Work out the finished part from the listing and answer in its coordinate system (mm). Face numbers are marked on the shaded views. A direction names the side the tool comes from. Coordinates: 2 decimals unless noted, no trailing zeros. Order: outer loops, then holes, each group sorted by start corner. A loop starts at its lowest first (then second) coordinate and runs counter-clockwise, first axis right, second up. Notation, with made-up numbers: M 78.25,-18.5 L 131.25,-18.5 A17 ccw 131.25,-3.5 Z; hole C -27,-6.75 d4. An arc over 180 degrees is marked long. Use a Markdown table: item, result.
from build123d import *

# Parameters (mm, degrees)
F0_W     = 430
F0_H     = 80
F1_DEPTH = 40
F2_W     = 7
F2_H     = 17.641502
F3_DEPTH = 30


with BuildPart() as f1:
    # F0 (on Right) → F1 (new body, symmetric)
    with BuildSketch(Plane.YZ):
        Rectangle(F0_W, F0_H)
    extrude(amount=F1_DEPTH, both=True)

    # F2 (on Right) → F3 (cut, symmetric)
    with BuildSketch(Plane.YZ):
        with Locations((-88.5, -48.820751)):
            Rectangle(F2_W, F2_H)
        Polygon((-92, -40), (-85, -40), (-17.87203, 40), (-17.87203, 50), (-106.093367, 50), (-106.093367, 40), (-87.336923, -30), align=None)
    extrude(amount=F3_DEPTH, both=True, mode=Mode.SUBTRACT)


solid = f1.part
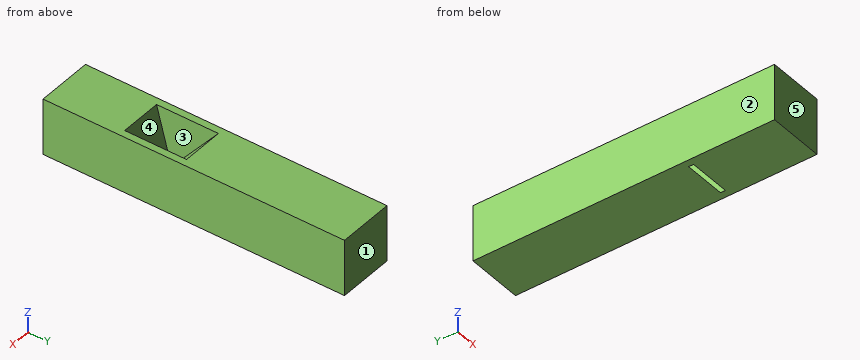
1. Section A-A on x = 12 is taken. Determine the outline of the cut face in (y, z), then the cut area to 3 significant figures.
Answers below:
| item | result |
|---|---|
| outline | M -215,-40 L -92,-40 L -87.34,-30 L -106.09,40 L -215,40 Z; M -85,-40 L 215,-40 L 215,40 L -17.87,40 Z |
| area | 30,800 mm² |
2. Find the intervals of material crossed by probe 1 along X at (y, z) = (-50.5, 8.5); probe 2 along Y at (x, z) = (-13, -10); probe 3 along Y at (x, z) = (16, 25.5), in increasing order.
Answers below:
| item | result |
|---|---|
| probe 1 | -40 to -30, 30 to 40 |
| probe 2 | -215 to -92.7, -59.83 to 215 |
| probe 3 | -215 to -102.21, -30.04 to 215 |
3. Section C-C on y = -97.5 is taken. Determine the outline of the cut face in (x, z), then the cut area to 3 significant figures.
Answers below:
| item | result |
|---|---|
| outline | M -40,-40 L 40,-40 L 40,40 L 30,40 L 30,7.93 L -30,7.93 L -30,40 L -40,40 Z |
| area | 4,480 mm² |
4. For the marked faces 4 and 5, determine the directions among +Z, -Z, +X, -X, +Y, -Y from which every point of the face is accessible in a straight line to the end or side of a thin tool.
Answers below:
| item | result |
|---|---|
| face 4 | +Z |
| face 5 | +Z, -Z, +X, -X, -Y |
5. For a pull along X with two mould halves and no side action, classify the marked faces 1, 2 and 3 as +X half, -X half, draft (parallel to the pull), parting line (faces both ways), or undercut.
Answers below:
| item | result |
|---|---|
| face 1 | draft |
| face 2 | -X half |
| face 3 | undercut |
6. Section D-D on z = -24 is taken. Determine the outline of the cut face in (x, y), then the cut area to 3 significant figures.
Answers below:
| item | result |
|---|---|
| outline | M -40,-215 L 40,-215 L 40,215 L -40,215 Z; hole M -30,-88.94 L 30,-88.94 L 30,-71.57 L -30,-71.57 Z |
| area | 33,400 mm² |
7. Section B-B on z = 26 is taken. Determine the outline of the cut face in (x, y), then the cut area to 3 significant figures.
Answers below:
| item | result |
|---|---|
| outline | M -40,-215 L 40,-215 L 40,215 L -40,215 Z; hole M -30,-102.34 L 30,-102.34 L 30,-29.62 L -30,-29.62 Z |
| area | 30,000 mm² |
